from build123d import *

# Parameters (mm, degrees)
SKETCH_3_W          = 29
SKETCH_3_H          = 95
EXTRUDE_1_DEPTH     = 40
SKETCH_4_R          = 3.005
CUT_EXTRUDE_1_DEPTH = 108.079409785
SKETCH_6_W          = 40
SKETCH_6_H          = 15
EXTRUDE_3_DEPTH     = 30
SKETCH_7_W          = 14.5
SKETCH_7_H          = 65
CUT_EXTRUDE_2_DEPTH = 108.354552768
SKETCH_9_R          = 2
CUT_EXTRUDE_4_DEPTH = 5
SKETCH_10_R         = 2
CUT_EXTRUDE_5_DEPTH = 5
SKETCH_11_R         = 2
CUT_EXTRUDE_6_DEPTH = 5
SKETCH_12_R         = 2
CUT_EXTRUDE_7_DEPTH = 5


with BuildPart() as part:
    # 草图3 → 凸台-拉伸1 (new body)
    with BuildSketch(Plane.XY):
        with Locations((14.5, 47.5)):
            Rectangle(SKETCH_3_W, SKETCH_3_H)
    extrude(amount=EXTRUDE_1_DEPTH)

    # 草图4 → 切除-拉伸1 (cut, through all)
    with BuildSketch(Plane.XY.offset(40)):
        with Locations((14.5, 52)):
            Circle(SKETCH_4_R)
        with Locations((14.5, 18)):
            Circle(SKETCH_4_R)
    extrude(amount=-CUT_EXTRUDE_1_DEPTH, mode=Mode.SUBTRACT)

    # 草图6 → 凸台-拉伸3 (add)
    with BuildSketch(Plane.ZY):
        with Locations((20, 87.5)):
            Rectangle(SKETCH_6_W, SKETCH_6_H)
    extrude(amount=EXTRUDE_3_DEPTH)

    # 草图7 → 切除-拉伸2 (cut, through all)
    with BuildSketch(Plane.XY.offset(40)):
        with Locations((7.25, 32.5)):
            Rectangle(SKETCH_7_W, SKETCH_7_H)
    extrude(amount=-CUT_EXTRUDE_2_DEPTH, mode=Mode.SUBTRACT)

    # 草图9 → 切除-拉伸4 (cut)
    with BuildSketch(Plane.ZY.offset(-14.5)):
        with Locations(Location((5, 60.0025, 0), (0, 0, 270))):
            Circle(SKETCH_9_R)
        with Locations(Location((35, 60.0025, 0), (0, 0, 270))):
            Circle(SKETCH_9_R)
    extrude(amount=-CUT_EXTRUDE_4_DEPTH, mode=Mode.SUBTRACT)

    # 草图10 → 切除-拉伸5 (cut)
    with BuildSketch(Plane.ZY.offset(-14.5)):
        with Locations(Location((5, 7.4975, 0), (0, 0, 270))):
            Circle(SKETCH_10_R)
        with Locations(Location((35, 7.4975, 0), (0, 0, 270))):
            Circle(SKETCH_10_R)
    extrude(amount=-CUT_EXTRUDE_5_DEPTH, mode=Mode.SUBTRACT)

    # 草图11 → 切除-拉伸6 (cut)
    with BuildSketch(Plane.ZY.offset(-14.5)):
        with Locations(Location((5, 35, 0), (0, 0, 270))):
            Circle(SKETCH_11_R)
        with Locations(Location((35, 35, 0), (0, 0, 270))):
            Circle(SKETCH_11_R)
    extrude(amount=-CUT_EXTRUDE_6_DEPTH, mode=Mode.SUBTRACT)

    # 草图12 → 切除-拉伸7 (cut)
    with BuildSketch(Plane(origin=(0, 95, 0), x_dir=(1, 0, 0), z_dir=(0, 1, 0))):
        with Locations(Location((-25, -35.563533882, 0), (0, 0, 270))):
            Circle(SKETCH_12_R)
        with Locations(Location((-25, -5.563533882, 0), (0, 0, 270))):
            Circle(SKETCH_12_R)
    extrude(amount=-CUT_EXTRUDE_7_DEPTH, mode=Mode.SUBTRACT)


solid = part.part
Could you check a few things on this model? Use its own coordinates, in mm. A direction names the side the tool comes from. Coordinates: 2 decimals unless noted, no trailing zeros. Loops run counter-clockwise (first coordinate to the right, second up) from the corner with the lowest first, then second, coordinate; pieces in that order, holes last.
1. Imagine slicing it at C-C (z = 35). Please give me the cut outline in (x, y) (1 decimal), and give its area (3 significant figures).
2. Imagine slicing it at B-B (y = 35). Please give me the cut outline in (x, z).
3. We'd pull the mould along Y, two halves only. Please class faces 1 (the face through (-25, 90, 36)), 2 (the face through (14.5, 60, 20)), 3 (the face through (17, 61.6, 33.8)): released by +Y, released by -Y, zero draft, split by the parting line, or undercut.
4. Imagine slicing it at D-D (y = 56). Please give me the cut outline in (x, z), and give its area (3 significant figures).
5. Imagine slicing it at A-A (x = -25). Please give me the cut outline in (y, z).
6. For faces 4 (the face through (19.5, 35, 35)), 5 (the face through (-25.77, 92.54, 37.41)), 6 (the face through (0, 72, 20)), which set-ups out of +Z, -Z, +X, -X, +Y, -Y let a thin tool reach every point of the face, with its end or its side?
7. For P1, Ø3, axis at y = 62, z = 21, coming from the -X side; P2, Ø16.5, axis at y = 69, z = 30, coming from the -X side; P3, Ø3, axis at y = 35, z = 35, coming from the -X side, each with a flat end and sliding along its axis, tell me the tip position at first contact or that it passes through.
8. I need wall thicknesses on L1, parallel to Y at x = 17, z = 11; L2, parallel to Y at x = 16, z = 24.5; L3, parallel to Y at x = 2, z = 33. Which ranges of each line are inside material? Lowest first, please.
Computed values:
1. outline: (-30, 80) - (0, 80) - (0, 65) - (14.5, 65) - (14.5, 62) - (19.5, 62) - (19.5, 58) - (14.5, 58) - (14.5, 55) arc R3 cw to (14.5, 49) - (14.5, 37) - (19.5, 37) - (19.5, 33) - (14.5, 33) - (14.5, 21) arc R3 cw to (14.5, 15) - (14.5, 9.5) - (19.5, 9.5) - (19.5, 5.5) - (14.5, 5.5) - (14.5, 0) - (29, 0) - (29, 95) - (-23.1, 95) - (-23.1, 90) - (-26.9, 90) - (-26.9, 95) - (-30, 95) - close
1. area: 2,150 mm2
2. outline: (14.5, 0) - (29, 0) - (29, 40) - (14.5, 40) - (14.5, 37) - (19.5, 37) - (19.5, 33) - (14.5, 33) - (14.5, 7) - (19.5, 7) - (19.5, 3) - (14.5, 3) - close
3. face 1: released by +Y
3. face 2: zero draft
3. face 3: undercut
4. outline: (14.5, 0) - (29, 0) - (29, 40) - (14.5, 40) - close
4. area: 580 mm2
5. outline: (80, 0) - (95, 0) - (95, 3.56) - (90, 3.56) - (90, 7.56) - (95, 7.56) - (95, 33.56) - (90, 33.56) - (90, 37.56) - (95, 37.56) - (95, 40) - (80, 40) - close
6. face 4: -X
6. face 5: +Y
6. face 6: +Z, -Z, -X, -Y
7. P1: stops at x = 14.5
7. P2: stops at x = 0
7. P3: stops at x = 19.5
8. L1: y = 0 to 16.33, 19.67 to 50.33, 53.67 to 95
8. L2: y = 0 to 15.4, 20.6 to 49.4, 54.6 to 95
8. L3: y = 65 to 95
